from build123d import *

# Parameters (mm, degrees)
SKETCH_1_R      = 1.5
EXTRUDE_2_DEPTH = 3
EXTRUDE_4_DEPTH = 3
EXTRUDE_6_DEPTH = 3


with BuildPart() as part:
    # 草圖1 → 填料-伸長2 (new body)
    with BuildSketch(Plane.XY):
        with BuildLine():
            Line((-1.793397634, 8.819508202), (-1.677039065, 11.819508202))
            ThreePointArc((-1.677039065, 11.819508202), (-1.118204833, 12.784789062), (-0.06994368, 13.165855188))
            Line((-0.06994368, 13.165855188), (0.06994368, 13.165855188))
            ThreePointArc((0.06994368, 13.165855188), (1.118204833, 12.784789062), (1.677039065, 11.819508202))
            Line((1.677039065, 11.819508202), (1.793397634, 8.819508202))
            ThreePointArc((1.793397634, 8.819508202), (2.781152949, 8.559508647), (3.73308769, 8.189264698))
            Line((3.73308769, 8.189264698), (5.590579507, 10.54792183))
            ThreePointArc((5.590579507, 10.54792183), (6.610063751, 11.000375931), (7.682109887, 10.692512456))
            Line((7.682109887, 10.692512456), (7.795281139, 10.610288729))
            ThreePointArc((7.795281139, 10.610288729), (8.419357178, 9.685847311), (8.304085714, 8.576444171))
            Line((8.304085714, 8.576444171), (6.634866017, 6.080999337))
            ThreePointArc((6.634866017, 6.080999337), (7.281152949, 5.290067271), (7.8336604, 4.431000423))
            Line((7.8336604, 4.431000423), (10.722786724, 5.24738783))
            ThreePointArc((10.722786724, 5.24738783), (11.81351265, 5.014193083), (12.499858583, 4.134993391))
            Line((12.499858583, 4.134993391), (12.543086154, 4.001952606))
            ThreePointArc((12.543086154, 4.001952606), (12.504601244, 2.887241097), (11.759253866, 2.057469969))
            Line((11.759253866, 2.057469969), (8.942041093, 1.01975541))
            ThreePointArc((8.942041093, 1.01975541), (9, 0), (8.942041093, -1.01975541))
            Line((8.942041093, -1.01975541), (11.759253866, -2.057469969))
            ThreePointArc((11.759253866, -2.057469969), (12.504601244, -2.887241097), (12.543086154, -4.001952606))
            Line((12.543086154, -4.001952606), (12.499858583, -4.134993391))
            ThreePointArc((12.499858583, -4.134993391), (11.81351265, -5.014193083), (10.722786724, -5.24738783))
            Line((10.722786724, -5.24738783), (7.8336604, -4.431000423))
            ThreePointArc((7.8336604, -4.431000423), (7.281152949, -5.290067271), (6.634866017, -6.080999337))
            Line((6.634866017, -6.080999337), (8.304085714, -8.576444171))
            ThreePointArc((8.304085714, -8.576444171), (8.419357178, -9.685847311), (7.795281139, -10.610288729))
            Line((7.795281139, -10.610288729), (7.682109887, -10.692512456))
            ThreePointArc((7.682109887, -10.692512456), (6.610063751, -11.000375931), (5.590579507, -10.54792183))
            Line((5.590579507, -10.54792183), (3.73308769, -8.189264698))
            ThreePointArc((3.73308769, -8.189264698), (2.781152949, -8.559508647), (1.793397634, -8.819508202))
            Line((1.793397634, -8.819508202), (1.677039065, -11.819508202))
            ThreePointArc((1.677039065, -11.819508202), (1.118204833, -12.784789062), (0.06994368, -13.165855188))
            Line((0.06994368, -13.165855188), (-0.06994368, -13.165855188))
            ThreePointArc((-0.06994368, -13.165855188), (-1.118204833, -12.784789062), (-1.677039065, -11.819508202))
            Line((-1.677039065, -11.819508202), (-1.793397634, -8.819508202))
            ThreePointArc((-1.793397634, -8.819508202), (-2.781152949, -8.559508647), (-3.73308769, -8.189264698))
            Line((-3.73308769, -8.189264698), (-5.590579507, -10.54792183))
            ThreePointArc((-5.590579507, -10.54792183), (-6.610063751, -11.000375931), (-7.682109887, -10.692512456))
            Line((-7.682109887, -10.692512456), (-7.795281139, -10.610288729))
            ThreePointArc((-7.795281139, -10.610288729), (-8.419357178, -9.685847311), (-8.304085714, -8.576444171))
            Line((-8.304085714, -8.576444171), (-6.634866017, -6.080999337))
            ThreePointArc((-6.634866017, -6.080999337), (-7.281152949, -5.290067271), (-7.8336604, -4.431000423))
            Line((-7.8336604, -4.431000423), (-10.722786724, -5.24738783))
            ThreePointArc((-10.722786724, -5.24738783), (-11.81351265, -5.014193083), (-12.499858583, -4.134993391))
            Line((-12.499858583, -4.134993391), (-12.543086154, -4.001952606))
            ThreePointArc((-12.543086154, -4.001952606), (-12.504601244, -2.887241097), (-11.759253866, -2.057469969))
            Line((-11.759253866, -2.057469969), (-8.942041093, -1.01975541))
            ThreePointArc((-8.942041093, -1.01975541), (-9, 0), (-8.942041093, 1.01975541))
            Line((-8.942041093, 1.01975541), (-11.759253866, 2.057469969))
            ThreePointArc((-11.759253866, 2.057469969), (-12.504601244, 2.887241097), (-12.543086154, 4.001952606))
            Line((-12.543086154, 4.001952606), (-12.499858583, 4.134993391))
            ThreePointArc((-12.499858583, 4.134993391), (-11.81351265, 5.014193083), (-10.722786724, 5.24738783))
            Line((-10.722786724, 5.24738783), (-7.8336604, 4.431000423))
            ThreePointArc((-7.8336604, 4.431000423), (-7.281152949, 5.290067271), (-6.634866017, 6.080999337))
            Line((-6.634866017, 6.080999337), (-8.304085714, 8.576444171))
            ThreePointArc((-8.304085714, 8.576444171), (-8.419357178, 9.685847311), (-7.795281139, 10.610288729))
            Line((-7.795281139, 10.610288729), (-7.682109887, 10.692512456))
            ThreePointArc((-7.682109887, 10.692512456), (-6.610063751, 11.000375931), (-5.590579507, 10.54792183))
            Line((-5.590579507, 10.54792183), (-3.73308769, 8.189264698))
            ThreePointArc((-3.73308769, 8.189264698), (-2.781152949, 8.559508647), (-1.793397634, 8.819508202))
        make_face()
        Circle(SKETCH_1_R, mode=Mode.SUBTRACT)
    extrude(amount=EXTRUDE_2_DEPTH)

    # 草圖2 → 填料-伸長4 (add)
    with BuildSketch(Plane.XY):
        with BuildLine():
            Line((0.06994368, 13.165855188), (0.06994368, 2.180013358))
            Line((0.06994368, 2.180013358), (-12.493626598, 4.153784946))
            ThreePointArc((-12.493626598, 4.153784946), (-7.674068466, 10.698285289), (0.06994368, 13.165855188))
        make_face()
    extrude(amount=EXTRUDE_4_DEPTH)

    # 草圖5 → 填料-伸長6 (add)
    with BuildSketch(Plane(origin=(0, 0, 0), x_dir=(-1, 0, 0), z_dir=(0, 0, -1))):
        Polygon((5.459056235, 11.60527133), (26.890281071, 32.301164585), (34.5983103, 71.955537312), (25.812503152, 97.136016411), (29.376125038, 106.046106934), (41.565268435, 71.111528315), (33.340538439, 28.798960582), (10.321664828, 6.569892728), align=None)
    extrude(amount=-EXTRUDE_6_DEPTH)


solid = part.part
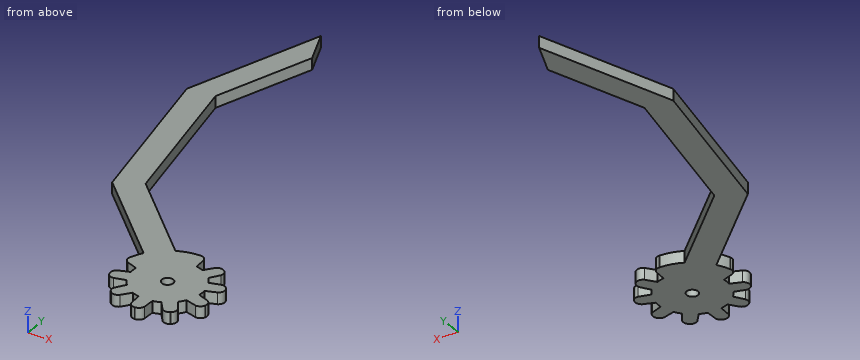
The model under review builds one solid part; all positions refer to its coordinate system, in mm. Round coordinates to 2 decimals unless told otherwise and drop trailing zeros. Loops run counter-clockwise (first coordinate to the right, second up) from the corner with the lowest first, then second, coordinate; pieces in that order, holes last. Notation, with made-up numbers: (65, 86) -> (75, 86) arc R23 cw to (75, 101) -> close; hole circle Ø11 at (63, 20). An arc over 180 degrees is marked (long way). Write item = value, one per line. Start each with the question number.
Item 1: Take a section at A-A on x = -21.5. Give the boundary of the cut face in (y, z), plus the area to 3 significant figures.
Item 2: Insertion check: pin 1 (1.8 mm diameter, centred on x = 0, y = 0, fed in from +Z); pin 2 (1.5 mm diameter, centred on x = 6, z = 0.5, fed in from +Y); pin 3 (1 mm diameter, centred on y = 79, z = 2, fed in from +X). Each pin has a flat end and moves straight along its axis. Give the tip position at first contact, or say it passes through.
Item 3: Take a section at B-B on y = 93. Give the boundary of the cut face in (x, z), plus the area to 3 significant figures.
Item 4: To check wall thickness, follow L1, parallel to Y at x = 0, z = 1.65; L2, parallel to Y at x = -8, z = 0.45; L3, parallel to X at y = 35, z = 0.6. State the ranges of each line that lie inside material, in increasing order.
Result:
q1.outline = (17.36, 0) -> (27.1, 0) -> (27.1, 3) -> (17.36, 3) -> close
q1.area = 29.2 mm²
q2.pin_1 = through
q2.pin_2 = 11
q2.pin_3 = -31.97
q3.outline = (-33.93, 0) -> (-27.26, 0) -> (-27.26, 3) -> (-33.93, 3) -> close
q3.area = 20.0 mm²
q4.L1 = -13.17 to -1.5, 1.5 to 13.17
q4.L2 = -10.43 to -8.12, -4.48 to 14.06
q4.L3 = -34.55 to -27.41
